```python
from build123d import *

# Parameters (mm, degrees)
BOSS_EXTRUDE1_DEPTH = 10


with BuildPart() as part:
    # Sketch1 → Boss-Extrude1 (new body)
    with BuildSketch(Plane(origin=(0, 0, 0), x_dir=(0, 0, -1), z_dir=(1, 0, 0))):
        Polygon((-84.5, 0), (84.5, 0), (103.022719545, 23.837300471), (85.030260907, 34.310612808), (68.481056011, 34.310612808), (90.006488303, 21.780775717), (82.690523765, 15.385421213), (60.999669369, 18.014714385), (24.911453349, 26.273949517), (41.001886779, 34.121778265), (-38.005922344, 79.73695813), (-83.198729811, 25), (-41.198729811, 25), align=None)
        Polygon((-47.179491924, 10), (-7.44944599, 10), (29.988283091, 10), (65.756507922, 10), (-10.545839316, 20.106291787), (19.714317813, 34.865156554), (1.503401285, 45.379234114), (-36.387555456, 67.255588188), (-62.314964122, 35), (-3.878221735, 35), (-18.992184521, 26.273949517), align=None, mode=Mode.SUBTRACT)
    extrude(amount=BOSS_EXTRUDE1_DEPTH)


solid = part.part
```
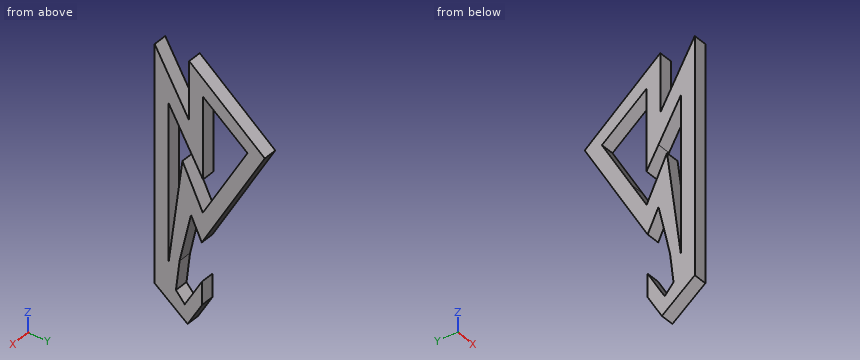
Could you check a few things on this model? Use its own coordinates, in mm. Coordinates: 2 decimals unless noted, no trailing zeros. Write each loop counter-clockwise with the first axis right and the second up, starting at its lowest first coordinate (ties: lowest second). Pieces come first, ordered by that corner, then holes. Notation, with made-up numbers: (62, -16.75) - (102, -16.75) arc R10 cw to (102, -1.75) - close; hole circle Ø11 at (6.25, 13). An arc over 180 degrees is marked (long way). Use a Markdown table: item, result.
Q1. Please list where these lines run through material, in increasing order: L1, parallel to Z at x = 0.5, y = 32.5; L2, parallel to Y at x = 6.5, z = 32.5; L3, parallel to Y at x = 4.75, z = 17.5.
Geometry check:
| item | result |
|---|---|
| L1 | z = -88.14 to -71.59, -37.68 to -14.87, 8.21 to 77.01 |
| L2 | y = 0 to 10, 18.48 to 35, 65.01 to 76.56 |
| L3 | y = 0 to 10, 27.14 to 35, 56.35 to 67.9 |
Q2. Imagine slicing it at D-D (z = 32). List the corners of the cut face in (x, y) for me, and give its area (3 significant figures).
Geometry check:
| item | result |
|---|---|
| outline | (0, 0) - (10, 0) - (10, 10) - (0, 10) - close; (0, 18.76) - (10, 18.76) - (10, 35) - (0, 35) - close; (0, 64.72) - (10, 64.72) - (10, 76.27) - (0, 76.27) - close |
| area | 378 mm2 |
Q3. I'm going to push flat-ended pins straight in: pin 1 Ø5 at (x, z) = (6.5, -80.5) entering from +Y; pin 2 Ø4 at (x, y) = (8, 57) entering from -Z; pin 3 Ø2 at (x, y) = (8.5, 18) entering from +Z; pin 4 Ø12 at (y, z) = (55.5, 29.5) entering from +X. Where does each tip first touch, or does it pass through?
Geometry check:
| item | result |
|---|---|
| pin 1 | stops at y = 34.31 |
| pin 2 | stops at z = -4.84 |
| pin 3 | stops at z = 55.06 |
| pin 4 | passes through |
Q4. Imagine slicing it at A-A (z = -37). List the corners of the cut face in (x, y) for me.
Geometry check:
| item | result |
|---|---|
| outline | (0, 0) - (10, 0) - (10, 10) - (0, 10) - close; (0, 13.81) - (10, 13.81) - (10, 23.51) - (0, 23.51) - close; (0, 32.17) - (10, 32.17) - (10, 36.43) - (0, 36.43) - close |
Q5. Imagine slicing it at B-B (x = 7.5). List the corners of the cut face in (y, z) for me, and give its area (3 significant figures).
Geometry check:
| item | result |
|---|---|
| outline | (0, -84.5) - (23.84, -103.02) - (34.31, -85.03) - (34.31, -68.48) - (21.78, -90.01) - (15.39, -82.69) - (18.01, -61) - (26.27, -24.91) - (34.12, -41) - (79.74, 38.01) - (25, 83.2) - (25, 41.2) - (0, 84.5) - close; hole (10, -65.76) - (20.11, 10.55) - (34.87, -19.71) - (67.26, 36.39) - (35, 62.31) - (35, 3.88) - (10, 47.18) - close |
| area | 5,130 mm2 |
Q6. Imagine slicing it at C-C (z = -78). List the corners of the cut face in (x, y) for me, and give its area (3 significant figures).
Geometry check:
| item | result |
|---|---|
| outline | (0, 0) - (10, 0) - (10, 15.95) - (0, 15.95) - close; (0, 28.77) - (10, 28.77) - (10, 34.31) - (0, 34.31) - close |
| area | 215 mm2 |
